```python
from build123d import *

# Parameters (mm, degrees)
BOSS_EXTRUDE1_DEPTH                                 = 5
SKETCH2_R                                           = 0.5
CUT_EXTRUDE1_DEPTH                                  = 44.011626335
CBORE_FOR_2_BINDING_HEAD_MACHINE_SCREW1_D           = 2.4384
CBORE_FOR_2_BINDING_HEAD_MACHINE_SCREW1_CBORE_D     = 5.55752
CBORE_FOR_2_BINDING_HEAD_MACHINE_SCREW1_CBORE_DEPTH = 2.499995
FILLET1_R                                           = 2
SKETCH6_R                                           = 4.35
CUT_EXTRUDE2_DEPTH                                  = 2
CBORE_FOR_M3_SBHCS1_D                               = 3.6
CBORE_FOR_M3_SBHCS1_CBORE_D                         = 6.7
CBORE_FOR_M3_SBHCS1_CBORE_DEPTH                     = 2.5


with BuildPart() as part:
    # Sketch1 → Boss-Extrude1 (new body)
    with BuildSketch(Plane(origin=(0, 0, 0), x_dir=(1, 0, 0), z_dir=(0, 1, 0))):
        with BuildLine():
            Line((-15, 0), (-15, 40))
            Line((-15, 40), (15, 40))
            Line((15, 40), (15, 0))
            ThreePointArc((15, 0), (0, -15), (-15, 0))
        make_face()
    extrude(amount=BOSS_EXTRUDE1_DEPTH)

    # Sketch2 → Cut-Extrude1 (cut, through all)
    with BuildSketch(Plane(origin=(0, 5, 0), x_dir=(1, 0, 0), z_dir=(0, 1, 0))):
        with Locations(Location((-8, 0, 0), (0, 0, 270))):
            Circle(SKETCH2_R)
        with Locations(Location((0, 9.5, 0), (0, 0, 270))):
            Circle(SKETCH2_R)
        with Locations(Location((8, 0, 0), (0, 0, 270))):
            Circle(SKETCH2_R)
        with Locations(Location((0, -9.5, 0), (0, 0, 270))):
            Circle(SKETCH2_R)
    extrude(amount=-CUT_EXTRUDE1_DEPTH, mode=Mode.SUBTRACT)

    # CBORE for #2 Binding Head Machine Screw1 (through all)
    with Locations(Plane(origin=(0, 0, 0), x_dir=(-1, 0, 0), z_dir=(0, -1, 0))):
        with Locations((-7.5, 35), (7.5, 35)):
            CounterBoreHole(CBORE_FOR_2_BINDING_HEAD_MACHINE_SCREW1_D / 2, CBORE_FOR_2_BINDING_HEAD_MACHINE_SCREW1_CBORE_D / 2, CBORE_FOR_2_BINDING_HEAD_MACHINE_SCREW1_CBORE_DEPTH)

    # Fillet1
    fillet1_edges = [part.edges().sort_by_distance(p)[0] for p in [
        (-15, 0, -20),
        (0, 0, -40),
        (15, 0, -20),
        (0, 0, 15),
        (-15, 2.5, -40),
        (15, 2.5, -40),
    ]]
    fillet(fillet1_edges, radius=FILLET1_R)

    # Sketch6 → Cut-Extrude2 (cut)
    with BuildSketch(Plane(origin=(0, 5, 0), x_dir=(1, 0, 0), z_dir=(0, 1, 0))):
        with Locations(Location((0, 0, 0), (0, 0, 270))):
            Circle(SKETCH6_R)
    extrude(amount=-CUT_EXTRUDE2_DEPTH, mode=Mode.SUBTRACT)

    # CBORE for M3 SBHCS1 (through all)
    with Locations(Plane(origin=(0, 0, 0), x_dir=(-1, 0, 0), z_dir=(0, -1, 0))):
        with Locations((0, 9.5), (8, 0), (0, -9.5), (-8, 0)):
            CounterBoreHole(CBORE_FOR_M3_SBHCS1_D / 2, CBORE_FOR_M3_SBHCS1_CBORE_D / 2, CBORE_FOR_M3_SBHCS1_CBORE_DEPTH)


solid = part.part
```
Read the model definition and answer for the solid it produces. Units are mm, in the model's axes. A direction names the side the tool comes from. Give positions to 0.01 mm unless a question says otherwise; leave off trailing zeros. Loops run counter-clockwise (first coordinate to the right, second up) from the corner with the lowest first, then second, coordinate; pieces in that order, holes last.
Item 1: The mould has two halves that part along Z. Classify faces 1 (the cylindrical face through (14.4, 3.52, -39.43)), 2 (the flat face through (6.6, 2.5, 1.4)), 3 (the cylindrical face through (0, 3, 15)), 4 (the flat face through (-15, 3, -19)): released by +Z, released by -Z, zero draft, split by the parting line, or undercut.
Item 2: Find the intervals of material crossed by line 1 along X through (y, z) = (0.6, -35); line 2 along X through (y, z) = (1.2, -35); line 3 along Z through (x, y) = (-6.5, 3.55), in increasing order.
Item 3: The part is cut by section B-B (x = 0). Write down the section's boundary in (y, z).
Item 4: For faces 5 (the cylindrical face through (-0.39, 3.768, -7.743)), 6 (the cylindrical face through (-2.65, 4.01, -3.45)), 7 (the flat face through (-9.4, 2.5, 1.4)), determine the directions among +Z, -Z, +X, -X, +Y, -Y from which every point of the face is accessible in a straight line to the end or side of a thin tool.
Item 5: Each of these flat-tipped pins is pushed along its axis until it touches: pin 1 Ø7 at (x, z) = (0.5, 2) entering from +Y; pin 2 Ø1 at (x, y) = (9.5, 4) entering from +Z; pin 3 Ø4 at (x, z) = (0, -9.5) entering from -Y. Where does it stop, or does it pass through?
Item 6: The part is cut by section A-A (z = -9.5). Write down the section's boundary in (x, y).
Item 7: The part is cut by section C-C (y = 4.2). Write down the section's boundary in (x, z).
Item 8: The part is cut by section D-D (x = -8). Give the number of separate pieces and of enclosed holes in the cut face, and give its area (3 significant figures).
Taken from the geometry:
1. face 1: released by -Z
1. face 2: undercut
1. face 3: released by +Z
1. face 4: zero draft
2. line 1: x = -14.43 to -10.28, -4.72 to 4.72, 10.28 to 14.43
2. line 2: x = -14.83 to -10.28, -4.72 to 4.72, 10.28 to 14.83
2. line 3: z = -40 to -35.7, -34.3 to -0.99, 0.99 to 13.52
3. outline: (0, -38) arc R2 ccw to (2, -40) - (5, -40) - (5, -11.3) - (2.5, -11.3) - (2.5, -12.85) - (0, -12.85) - close; (0, -6.15) - (2.5, -6.15) - (2.5, -7.7) - (5, -7.7) - (5, -4.35) - (3, -4.35) - (3, 4.35) - (5, 4.35) - (5, 7.7) - (2.5, 7.7) - (2.5, 6.15) - (0, 6.15) - close; (0, 12.85) - (2.5, 12.85) - (2.5, 11.3) - (5, 11.3) - (5, 15) - (2, 15) arc R2 ccw to (0, 13) - close
4. face 5: +Y, -Y
4. face 6: +Y
4. face 7: -Y
5. pin 1: stops at y = 5
5. pin 2: stops at z = 12
5. pin 3: stops at y = 2.5
6. outline: (-15, 2) arc R2 ccw to (-13, 0) - (-3.35, 0) - (-3.35, 2.5) - (-1.8, 2.5) - (-1.8, 5) - (-15, 5) - close; (1.8, 2.5) - (3.35, 2.5) - (3.35, 0) - (13, 0) arc R2 ccw to (15, 2) - (15, 5) - (1.8, 5) - close
7. outline: (-15, -38) arc R2 ccw to (-13, -40) - (13, -40) arc R2 ccw to (15, -38) - (15, 0) arc R15 ccw to (-15, 0) - close; hole circle Ø3.6 at (-8, 0); hole circle Ø2.44 at (-7.5, -35); hole circle Ø8.7 at (0, 0); hole circle Ø3.6 at (0, -9.5); hole circle Ø3.6 at (0, 9.5); hole circle Ø3.6 at (8, 0); hole circle Ø2.44 at (7.5, -35)
8. separate pieces: 3
8. enclosed holes: 0
8. area: 217 mm2
